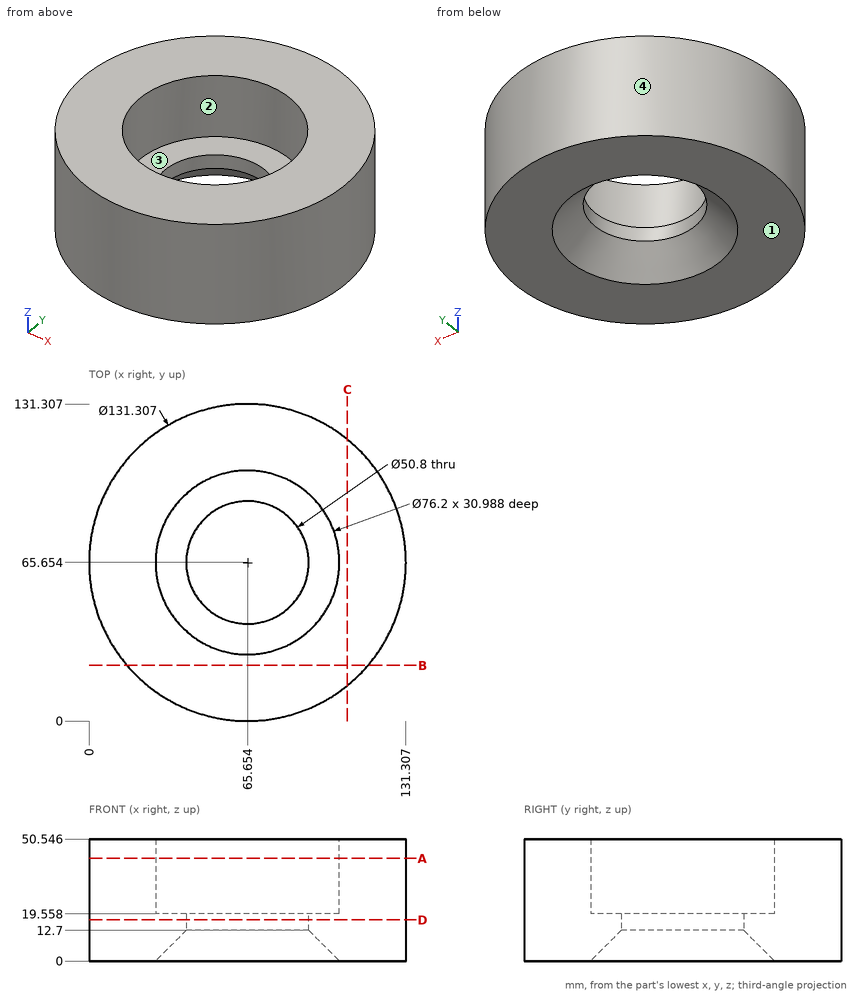
Answer from the drawing. Dimensions are ordinates in mm from the lowest x, y and z of the part. Give positions to 0.01 mm unless a question says otherwise; leave off trailing zeros. Loops run counter-clockwise (first coordinate to the right, second up) from the corner with the lowest first, then second, coordinate; pieces in that order, holes last. Notation, with made-up numbers: (33, 23.5) - (82, 23.5) arc R13 ccw to (82, 35.5) - close; hole circle Ø1 at (44, 57.25). An arc over 180 degrees is marked (long way). Answer as a JSON object with one key per item and string values.
1. A cutting plane is placed at D-D (z = 17). Write down the section's boundary in (x, y).
Determined:
{"outline": "circle Ø131.31 at (65.65, 65.65); hole circle Ø50.8 at (65.65, 65.65)"}
2. Find the intervals of material crossed by L1, parallel to X at y = 91, z = 36; L2, parallel to Y at x = 51.5, z = 36.5 (1 decimal); L3, parallel to Y at x = 40.5, z = 6 (1 decimal), in increasing order. Write a range as [from, to].
Determined:
{"L1": "[5.09, 37.21], [94.1, 126.22]", "L2": "[1.5, 30.3], [101, 129.8]", "L3": "[5, 45.7], [85.6, 126.3]"}
3. For a pull along X with two mould halves and no side action, classify the marked faces 1, 2, 3 and 4 as pulls with the +X half, pulls with the -X half, needs draft (parallel to the pull), parting line crosses it, or undercut.
Determined:
{"face 1": "needs draft", "face 2": "undercut", "face 3": "undercut", "face 4": "parting line crosses it"}
4. A cutting plane is placed at A-A (z = 42.5). Write down the section's boundary in (x, y), then the cut area to 3 significant figures.
Determined:
{"outline": "circle Ø131.31 at (65.65, 65.65); hole circle Ø76.2 at (65.65, 65.65)", "area": "8,980 mm²"}
5. Flat-ended cylindrical pins translate along their axes: pin 1 Ø6 at (x, z) = (58, 20) entering from +Y; pin 2 Ø4 at (y, z) = (15.5, 7.5) entering from -X (1 decimal); pin 3 Ø3 at (x, y) = (86.5, 38) entering from +Z. Find the tip coordinate at first contact, or state that the pin passes through.
Determined:
{"pin 1": "y = 131.14", "pin 2": "x = 21", "pin 3": "z = 19.56"}
6. A cutting plane is placed at C-C (x = 107). Write down the section's boundary in (y, z) (1 decimal).
Determined:
{"outline": "(14.7, 0) - (116.7, 0) - (116.7, 50.5) - (14.7, 50.5) - close"}
7. A cutting plane is placed at B-B (y = 23). Write down the section's boundary in (x, z) (1 decimal), then the cut area to 3 significant figures.
Determined:
{"outline": "(15.7, 0) - (115.6, 0) - (115.6, 50.5) - (15.7, 50.5) - close", "area": "5,050 mm²"}
